Build history of the part. All positions in model axes, mm. A direction names the side the tool comes from. Round coordinates to 2 decimals unless told otherwise and drop trailing zeros. Write each loop counter-clockwise with the first axis right and the second up, starting at its lowest first coordinate (ties: lowest second). Pieces come first, ordered by that corner, then holes. Notation, with made-up numbers: (29, 65) -> (64, 65) arc R13 cw to (64, 72) -> close; hole circle Ø6 at (-11, 19.5). An arc over 180 degrees is marked (long way). Answer in a Markdown table with one row per item.
```python
from build123d import *

# Parameters (mm, degrees)
F0_R     = 3.175
F1_DEPTH = 3.048


with BuildPart() as f1:
    # F0 (on Front) → F1 (new body)
    with BuildSketch(Plane.XZ):
        with BuildLine():
            ThreePointArc((-9.4589602313, 115.4196858236), (-0.5608158331, 104.7915242756), (9.525, 114.3))
            ThreePointArc((9.525, 114.3), (0.5608158331, 123.8084757244), (-9.4589602313, 115.4196858236))
        make_face()
        with Locations((0, 114.3)):
            Circle(F0_R, mode=Mode.SUBTRACT)
        with BuildLine():
            Line((15.3865384615, 67.4076923077), (9.525, 114.3))
            ThreePointArc((9.525, 114.3), (-0.5608158331, 104.7915242756), (-9.4589602313, 115.4196858236))
            Line((-9.4589602313, 115.4196858236), (-14.9842264132, 68.7429556358))
            ThreePointArc((-14.9842264132, 68.7429556358), (0.6972774089, 79.3596793541), (15.3865384615, 67.4076923077))
        make_face()
        with Locations((-3.175, 100.0252)):
            Circle(F0_R, mode=Mode.SUBTRACT)
        with BuildLine():
            Line((15.875, 63.5), (15.3865384615, 67.4076923077))
            ThreePointArc((15.3865384615, 67.4076923077), (0.6972774089, 79.3596793541), (-14.9842264132, 68.7429556358))
            Line((-14.9842264132, 68.7429556358), (-15.7942028036, 61.9003804205))
            ThreePointArc((-15.7942028036, 61.9003804205), (0.8008294116, 47.6452121662), (15.875, 63.5))
        make_face()
        with Locations((0, 63.5)):
            Circle(F0_R, mode=Mode.SUBTRACT)
        with BuildLine():
            ThreePointArc((15.875, 63.5), (15.7524112928, 65.4690514116), (15.3865384615, 67.4076923077))
            Line((15.3865384615, 67.4076923077), (15.875, 63.5))
        make_face()
        with BuildLine():
            Line((-15.7942028036, 61.9003804205), (-14.9842264132, 68.7429556358))
            ThreePointArc((-14.9842264132, 68.7429556358), (-15.7649337188, 65.3661430393), (-15.7942028036, 61.9003804205))
        make_face()
        with BuildLine():
            Line((15.875, 15.8877), (15.875, 63.5))
            ThreePointArc((15.875, 63.5), (0.8008294116, 47.6452121662), (-15.7942028036, 61.9003804205))
            Line((-15.7942028036, 61.9003804205), (-9.525, 0))
            ThreePointArc((-9.525, 0), (0, 9.525), (9.525, 0))
            ThreePointArc((9.525, 0), (6.854787681, -6.6134341191), (0.3412706881, -9.5188843526))
            Line((0.3412706881, -9.5188843526), (44.45, -7.9375))
            ThreePointArc((44.45, -7.9375), (36.5125, 0), (44.45, 7.9375))
            Line((44.45, 7.9375), (23.8252, 7.9375))
            ThreePointArc((23.8252, 7.9375), (18.2035596682, 10.2660596682), (15.875, 15.8877))
        make_face()
        with BuildLine():
            ThreePointArc((9.525, 0), (0, 9.525), (-9.525, 0))
            ThreePointArc((-9.525, 0), (-6.6134341191, -6.854787681), (0.3412706881, -9.5188843526))
            ThreePointArc((0.3412706881, -9.5188843526), (6.854787681, -6.6134341191), (9.525, 0))
        make_face()
        Circle(F0_R, mode=Mode.SUBTRACT)
        with BuildLine():
            ThreePointArc((52.3875, 0), (50.0626600757, 5.6126600757), (44.45, 7.9375))
            ThreePointArc((44.45, 7.9375), (36.5125, 0), (44.45, -7.9375))
            ThreePointArc((44.45, -7.9375), (50.0626600757, -5.6126600757), (52.3875, 0))
        make_face()
        with Locations((44.45, 0)):
            Circle(F0_R, mode=Mode.SUBTRACT)
    extrude(amount=F1_DEPTH)


solid = f1.part
```
Q1. Saw through at C-C on z = 52. Write the cut outline in (x, y) (1 decimal), plus the area to 3 significant figures.
A:
| item | result |
|---|---|
| outline | (-14.8, -3) -> (15.9, -3) -> (15.9, 0) -> (-14.8, 0) -> close |
| area | 93.5 mm² |
Q2. Two-plate mould, pull along Z, no slides. Class faces 3 (the cylindrical face through (0.762, -1.503, 123.794)), 4 (the flat face through (3, 0, 43)), 5 (the cylindrical face through (1.707, -1.503, 66.177)): released by +Z, released by -Z, zero draft, split by the parting line, or undercut.
A:
| item | result |
|---|---|
| face 3 | released by +Z |
| face 4 | zero draft |
| face 5 | undercut |
Q3. Which spindle directions (+Z, -Z, +X, -X, +Y, -Y) get a long thin tool onto all of the face, cutting with end or side? Do faces 1 (the cylindrical face through (-0.69, -1.5, 111.2)), 2 (the flat face through (15.875, -2, 39)). Say none if no direction does.
A:
| item | result |
|---|---|
| face 1 | +Y, -Y |
| face 2 | +Z, +X, +Y, -Y |
Q4. Wall check: line 1 (X direction, y = -1.2, z = -2); line 2 (X direction, y = -0.65, z = 102); line 3 (Z direction, x = 46, y = -1.65). Give the ranges that are in metal, low to high. Write a range as [from, to].
A:
| item | result |
|---|---|
| line 1 | [-9.31, -2.47], [2.47, 41.98], [46.92, 52.13] |
| line 2 | [-11.05, -5.66], [-0.69, 11.06] |
| line 3 | [-7.78, -2.77], [2.77, 7.78] |
Q5. Saw through at B-B on x = 22. Write the cut outline in (y, z).
A:
| item | result |
|---|---|
| outline | (-3.05, -8.74) -> (0, -8.74) -> (0, 8.15) -> (-3.05, 8.15) -> close |
Q6. Drop flat-ended pins along their axis: P1, Ø1.5, axis at x = 33, y = -1.5, coming from the +Z side; P2, Ø0.9, axis at y = -1.5, z = 47.5, coming from the +X side (3 decimals); P3, Ø1.5, axis at y = -2.5, z = 25, coming from the -X side. Give the stop position or say it passes through.
A:
| item | result |
|---|---|
| P1 | z = 7.94 |
| P2 | x = 15.875 |
| P3 | x = -12.13 |
Q7. Saw through at A-A on y = -0.65. State how many separate pieces and enclosed holes the cut face has, plus the area to 3 significant figures.
A:
| item | result |
|---|---|
| separate pieces | 1 |
| enclosed holes | 5 |
| area | 3,890 mm² |
